from build123d import *

# Parameters (mm, degrees)
SKETCH1_W              = 250
SKETCH1_H              = 300
BOSS_EXTRUDE1_DEPTH    = 2.38125
SKETCH2_W              = 20.2
SKETCH2_H              = 40.5
CUT_EXTRUDE1_DEPTH     = 3.38125
SKETCH3_R              = 2.25
CUT_EXTRUDE2_DEPTH     = 3.38125
FILLET1_R              = 0.5
LPATTERN1_COUNT        = 4
LPATTERN1_PITCH        = 62
FILLET1_OF_LPATTERN1_R = 0.5
SKETCH4_W              = 106
SKETCH4_H              = 68
CUT_EXTRUDE3_DEPTH     = 3.38125
SKETCH5_W              = 8
SKETCH5_H              = 5
SKETCH5_W_2            = 12
SKETCH5_H_2            = 27.5
CUT_EXTRUDE4_DEPTH     = 3.38125
FILLET2_R              = 0.25
SKETCH6_R              = 2
CUT_EXTRUDE5_DEPTH     = 3.38125
SKETCH7_R              = 2.25
CUT_EXTRUDE6_DEPTH     = 3.38125
FILLET3_R              = 2.5
CUT_EXTRUDE7_REACH     = 4.381
SKETCH8_R              = 2.25
CUT_EXTRUDE8_REACH     = 4.381
SKETCH9_R              = 2.5


with BuildPart() as part:
    # Sketch1 → Boss-Extrude1 (new body)
    with BuildSketch(Plane(origin=(0, 0, 0), x_dir=(1, 0, 0), z_dir=(0, 1, 0))):
        with Locations((125, 150)):
            Rectangle(SKETCH1_W, SKETCH1_H)
    extrude(amount=BOSS_EXTRUDE1_DEPTH)

    # Sketch2 → Cut-Extrude1 (cut, through all)
    with BuildSketch(Plane(origin=(0, 2.38125, 0), x_dir=(1, 0, 0), z_dir=(0, 1, 0))):
        with Locations((32, 129.75)):
            Rectangle(SKETCH2_W, SKETCH2_H)
    cut_extrude1 = extrude(amount=-CUT_EXTRUDE1_DEPTH, mode=Mode.SUBTRACT)

    # Sketch3 → Cut-Extrude2 (cut, through all)
    with BuildSketch(Plane(origin=(0, 2.38125, 0), x_dir=(1, 0, 0), z_dir=(0, 1, 0))):
        with Locations((37, 104.75)):
            Circle(SKETCH3_R)
        with Locations((27, 104.75)):
            Circle(SKETCH3_R)
        with BuildLine():
            Line((28, 157), (27, 157))
            ThreePointArc((27, 157), (24.80939278, 154.236443763), (28, 152.734435563))
            Line((28, 152.734435563), (28, 150))
            Line((28, 150), (36, 150))
            Line((36, 150), (36, 152.734435563))
            ThreePointArc((36, 152.734435563), (39.19060722, 154.236443763), (37, 157))
            Line((37, 157), (36, 157))
            Line((36, 157), (28, 157))
        make_face()
    cut_extrude2 = extrude(amount=-CUT_EXTRUDE2_DEPTH, mode=Mode.SUBTRACT)

    # Fillet1
    fillet1_edges = [part.edges().sort_by_distance(p)[0] for p in [
        (21.9, 1.190625, -109.5),
        (21.9, 1.190625, -150),
        (42.1, 1.190625, -150),
        (42.1, 1.190625, -109.5),
        (36, 1.190625, -152.734435563),
        (36, 1.190625, -150),
        (28, 1.190625, -150),
        (28, 1.190625, -152.734435563),
    ]]
    fillet(fillet1_edges, radius=FILLET1_R)

    # LPattern1: Cut-Extrude1, Cut-Extrude2 ×4
    with Locations(*[(i * LPATTERN1_PITCH, 0, 0) for i in range(1, LPATTERN1_COUNT)]):
        add(cut_extrude1, mode=Mode.SUBTRACT)
        add(cut_extrude2, mode=Mode.SUBTRACT)

    # Fillet1 of LPattern1
    fillet1_of_lpattern1_edges = [part.edges().sort_by_distance(p)[0] for p in [
        (83.9, 1.190625, -109.5),
        (83.9, 1.190625, -150),
        (104.1, 1.190625, -150),
        (104.1, 1.190625, -109.5),
        (98, 1.190625, -152.734435563),
        (98, 1.190625, -150),
        (90, 1.190625, -150),
        (90, 1.190625, -152.734435563),
        (145.9, 1.190625, -109.5),
        (145.9, 1.190625, -150),
        (166.1, 1.190625, -150),
        (166.1, 1.190625, -109.5),
        (160, 1.190625, -152.734435563),
        (160, 1.190625, -150),
        (152, 1.190625, -150),
        (152, 1.190625, -152.734435563),
        (207.9, 1.190625, -109.5),
        (207.9, 1.190625, -150),
        (228.1, 1.190625, -150),
        (228.1, 1.190625, -109.5),
        (222, 1.190625, -152.734435563),
        (222, 1.190625, -150),
        (214, 1.190625, -150),
        (214, 1.190625, -152.734435563),
    ]]
    fillet(fillet1_of_lpattern1_edges, radius=FILLET1_OF_LPATTERN1_R)

    # Sketch4 → Cut-Extrude3 (cut, through all)
    with BuildSketch(Plane(origin=(0, 2.38125, 0), x_dir=(1, 0, 0), z_dir=(0, 1, 0))):
        with Locations((117, 49)):
            Rectangle(SKETCH4_W, SKETCH4_H)
    extrude(amount=-CUT_EXTRUDE3_DEPTH, mode=Mode.SUBTRACT)

    # Sketch5 → Cut-Extrude4 (cut, through all)
    with BuildSketch(Plane(origin=(0, 2.38125, 0), x_dir=(1, 0, 0), z_dir=(0, 1, 0))):
        with Locations((196, 88.5)):
            Rectangle(SKETCH5_W, SKETCH5_H)
        with Locations((232, 88.5)):
            Rectangle(SKETCH5_W, SKETCH5_H)
        with Locations((32, 49)):
            Rectangle(SKETCH5_W_2, SKETCH5_H_2)
    extrude(amount=-CUT_EXTRUDE4_DEPTH, mode=Mode.SUBTRACT)

    # Fillet2
    fillet2_edges = [part.edges().sort_by_distance(p)[0] for p in [
        (64, 1.190625, -15),
        (64, 1.190625, -83),
        (170, 1.190625, -83),
        (170, 1.190625, -15),
        (26, 1.190625, -35.25),
        (26, 1.190625, -62.75),
        (38, 1.190625, -62.75),
        (38, 1.190625, -35.25),
        (228, 1.190625, -86),
        (228, 1.190625, -91),
        (236, 1.190625, -91),
        (236, 1.190625, -86),
        (192, 1.190625, -86),
        (192, 1.190625, -91),
        (200, 1.190625, -91),
        (200, 1.190625, -86),
    ]]
    fillet(fillet2_edges, radius=FILLET2_R)

    # Sketch6 → Cut-Extrude5 (cut, through all)
    with BuildSketch(Plane(origin=(0, 2.38125, 0), x_dir=(1, 0, 0), z_dir=(0, 1, 0))):
        with Locations((56, 85)):
            Circle(SKETCH6_R)
        with Locations((178, 85)):
            Circle(SKETCH6_R)
        with Locations((178, 13)):
            Circle(SKETCH6_R)
        with Locations((56, 13)):
            Circle(SKETCH6_R)
    extrude(amount=-CUT_EXTRUDE5_DEPTH, mode=Mode.SUBTRACT)

    # Sketch7 → Cut-Extrude6 (cut, through all)
    with BuildSketch(Plane(origin=(0, 2.38125, 0), x_dir=(1, 0, 0), z_dir=(0, 1, 0))):
        with Locations((10, 290)):
            Circle(SKETCH7_R)
        with Locations((240, 290)):
            Circle(SKETCH7_R)
        with Locations((240, 110)):
            Circle(SKETCH7_R)
        with Locations((240, 10)):
            Circle(SKETCH7_R)
        with Locations((10, 10)):
            Circle(SKETCH7_R)
        with Locations((10, 110)):
            Circle(SKETCH7_R)
    extrude(amount=-CUT_EXTRUDE6_DEPTH, mode=Mode.SUBTRACT)

    # Fillet3
    fillet3_edges = [part.edges().sort_by_distance(p)[0] for p in [
        (0, 1.190625, -300),
        (250, 1.190625, -300),
        (250, 1.190625, 0),
        (0, 1.190625, 0),
    ]]
    fillet(fillet3_edges, radius=FILLET3_R)

    # Sketch8 → Cut-Extrude7 (cut, up to next)
    with BuildSketch(Plane(origin=(0, 2.38125, 0), x_dir=(1, 0, 0), z_dir=(0, 1, 0)), mode=Mode.PRIVATE) as cut_extrude7_sk1:
        with Locations((214, 88.25)):
            Circle(SKETCH8_R)
    cut_extrude7_tool1 = extrude(cut_extrude7_sk1.sketch, amount=-CUT_EXTRUDE7_REACH, mode=Mode.PRIVATE) & part.part
    add(cut_extrude7_tool1.solids().sort_by_distance((214, 2.38125, -88.25))[0], mode=Mode.SUBTRACT)
    # Sketch8 → Cut-Extrude7 (cut, up to next)
    with BuildSketch(Plane(origin=(0, 2.38125, 0), x_dir=(1, 0, 0), z_dir=(0, 1, 0)), mode=Mode.PRIVATE) as cut_extrude7_sk2:
        with Locations((241.75, 50.5)):
            Circle(SKETCH8_R)
    cut_extrude7_tool2 = extrude(cut_extrude7_sk2.sketch, amount=-CUT_EXTRUDE7_REACH, mode=Mode.PRIVATE) & part.part
    add(cut_extrude7_tool2.solids().sort_by_distance((241.75, 2.38125, -50.5))[0], mode=Mode.SUBTRACT)
    # Sketch8 → Cut-Extrude7 (cut, up to next)
    with BuildSketch(Plane(origin=(0, 2.38125, 0), x_dir=(1, 0, 0), z_dir=(0, 1, 0)), mode=Mode.PRIVATE) as cut_extrude7_sk3:
        with Locations((214, 12.75)):
            Circle(SKETCH8_R)
    cut_extrude7_tool3 = extrude(cut_extrude7_sk3.sketch, amount=-CUT_EXTRUDE7_REACH, mode=Mode.PRIVATE) & part.part
    add(cut_extrude7_tool3.solids().sort_by_distance((214, 2.38125, -12.75))[0], mode=Mode.SUBTRACT)
    # Sketch8 → Cut-Extrude7 (cut, up to next)
    with BuildSketch(Plane(origin=(0, 2.38125, 0), x_dir=(1, 0, 0), z_dir=(0, 1, 0)), mode=Mode.PRIVATE) as cut_extrude7_sk4:
        with Locations((186.25, 50.5)):
            Circle(SKETCH8_R)
    cut_extrude7_tool4 = extrude(cut_extrude7_sk4.sketch, amount=-CUT_EXTRUDE7_REACH, mode=Mode.PRIVATE) & part.part
    add(cut_extrude7_tool4.solids().sort_by_distance((186.25, 2.38125, -50.5))[0], mode=Mode.SUBTRACT)

    # Sketch9 → Cut-Extrude8 (cut, up to next)
    with BuildSketch(Plane(origin=(0, 2.38125, 0), x_dir=(1, 0, 0), z_dir=(0, 1, 0)), mode=Mode.PRIVATE) as cut_extrude8_sk1:
        with Locations((32, 84.75)):
            Circle(SKETCH9_R)
    cut_extrude8_tool1 = extrude(cut_extrude8_sk1.sketch, amount=-CUT_EXTRUDE8_REACH, mode=Mode.PRIVATE) & part.part
    add(cut_extrude8_tool1.solids().sort_by_distance((32, 2.38125, -84.75))[0], mode=Mode.SUBTRACT)


solid = part.part
Source: CAD feature listing. Evaluate the final solid. Frame: model axes, mm. Round coordinates to 2 decimals unless told otherwise and drop trailing zeros. Loops run counter-clockwise (first coordinate to the right, second up) from the corner with the lowest first, then second, coordinate; pieces in that order, holes last. Notation, with made-up numbers: (50, 64.5) - (99, 64.5) arc R16 ccw to (99, 71.5) - close; hole circle Ø11 at (-6.75, 56). An arc over 180 degrees is marked (long way). Write item = value, one per line. Start each with the question number.
(1) Section query A-A, the plane z = -74. Output: boundary loops of the cut face in (x, y), plus the area to 3 significant figures.
(2) Section query B-B, the plane x = 75.5. Output: boundary loops of the cut face in (y, z), plus the area to 3 significant figures.
(3) Section query C-C, the plane z = -120.5. Output: boundary loops of the cut face in (x, y), plus the area to 3 significant figures.
(4) Section query D-D, the plane y = 0.6. State how many separate pieces and enclosed holes the cut face has, plus the area to 3 significant figures.
(5) Ray query, line 1 along Z through (x, y) = (37, 1.6); line 2 along Z through (x, y) = (157, 1.7); line 3 along X through (y, z) = (1.35, -13). Return the intervals inside material, ascending. Write a range as from..to.
Conclusion:
q1.outline = (0, 0) - (64, 0) - (64, 2.38) - (0, 2.38) - close; (170, 0) - (250, 0) - (250, 2.38) - (170, 2.38) - close
q1.area = 343 mm2
q2.outline = (0, -300) - (2.38, -300) - (2.38, -83) - (0, -83) - close; (0, -15) - (2.38, -15) - (2.38, 0) - (0, 0) - close
q2.area = 552 mm2
q3.outline = (0, 0) - (21.9, 0) - (21.9, 2.38) - (0, 2.38) - close; (42.1, 0) - (83.9, 0) - (83.9, 2.38) - (42.1, 2.38) - close; (104.1, 0) - (145.9, 0) - (145.9, 2.38) - (104.1, 2.38) - close; (166.1, 0) - (207.9, 0) - (207.9, 2.38) - (166.1, 2.38) - close; (228.1, 0) - (250, 0) - (250, 2.38) - (228.1, 2.38) - close
q3.area = 403 mm2
q4.separate_pieces = 1
q4.enclosed_holes = 31
q4.area = 63,400 mm2
q5.line_1 = -300..-157, -152.5..-150, -109.5..-107, -102.5..-62.75, -35.25..0
q5.line_2 = -300..-157, -109.5..-83, -15..0
q5.line_3 = 0..54, 58..176, 180..211.76, 216.24..250
